```python
from build123d import *

# Parameters (mm, degrees)
SKETCH1_W           = 700
SKETCH1_H           = 50
SKETCH1_R           = 6
BOSS_EXTRUDE1_DEPTH = 10
FILLET1_RADIUS      = 25
FILLET1_LENGTH      = 10
FILLET2_RADIUS      = 25
FILLET2_LENGTH      = 10
BOSS_EXTRUDE2_DEPTH = 10
SKETCH3_R           = 100
SKETCH3_R_2         = 82.5
BOSS_EXTRUDE3_DEPTH = 30
SKETCH4_R           = 4.5
CUT_EXTRUDE1_DEPTH  = 815.631818676
CIRPATTERN1_COUNT   = 8


with BuildPart() as part:
    # Sketch1 → Boss-Extrude1 (new body)
    with BuildSketch(Plane.XY):
        Rectangle(SKETCH1_W, SKETCH1_H)
        with Locations((-300, 0)):
            Circle(SKETCH1_R, mode=Mode.SUBTRACT)
        with Locations((300, 0)):
            Circle(SKETCH1_R, mode=Mode.SUBTRACT)
    extrude(amount=BOSS_EXTRUDE1_DEPTH)

    # Fillet1: full round fillet: the end face becomes a half cylinder, R = half its width
    fillet1_face = Plane((-350, 0, 5), x_dir=(0, 0, 1), z_dir=(-1, 0, 0))  # on the end face: x along it, z out of the body
    fillet1_slab = fillet1_face.offset(-FILLET1_RADIUS / 2) * Box(FILLET1_LENGTH, 2 * FILLET1_RADIUS, FILLET1_RADIUS, mode=Mode.PRIVATE)  # the body's end, R deep
    fillet1_round = Plane((-325, 0, 5), x_dir=(-1, 0, 0), z_dir=(0, 0, 1)) * Cylinder(FILLET1_RADIUS, FILLET1_LENGTH, mode=Mode.PRIVATE)  # its axis R under the face
    add(fillet1_slab - fillet1_round, mode=Mode.SUBTRACT)

    # Fillet2: full round fillet: the end face becomes a half cylinder, R = half its width
    fillet2_face = Plane((350, 0, 5), x_dir=(0, 0, -1), z_dir=(1, 0, 0))  # on the end face: x along it, z out of the body
    fillet2_slab = fillet2_face.offset(-FILLET2_RADIUS / 2) * Box(FILLET2_LENGTH, 2 * FILLET2_RADIUS, FILLET2_RADIUS, mode=Mode.PRIVATE)  # the body's end, R deep
    fillet2_round = Plane((325, 0, 5), x_dir=(1, 0, 0), z_dir=(0, 0, -1)) * Cylinder(FILLET2_RADIUS, FILLET2_LENGTH, mode=Mode.PRIVATE)  # its axis R under the face
    add(fillet2_slab - fillet2_round, mode=Mode.SUBTRACT)

    # Sketch2 → Boss-Extrude2 (add)
    with BuildSketch(Plane.XY.offset(10)):
        Polygon((-325, 25), (-85, 735), (85, 735), (325, 25), align=None)
    extrude(amount=-BOSS_EXTRUDE2_DEPTH)

    # Sketch3 → Boss-Extrude3 (add)
    with BuildSketch(Plane.XY.offset(10)):
        with Locations(Location((0, 472, 0), (0, 0, 180))):
            Circle(SKETCH3_R)
        with Locations((0, 472)):
            Circle(SKETCH3_R_2, mode=Mode.SUBTRACT)
    extrude(amount=BOSS_EXTRUDE3_DEPTH)

    # Sketch4 → Cut-Extrude1 (cut, through all)
    with BuildSketch(Plane.XY.offset(10)):
        with Locations((-37.739196917, 413.044482735)):
            Circle(SKETCH4_R)
    cut_extrude1 = extrude(amount=-CUT_EXTRUDE1_DEPTH, mode=Mode.SUBTRACT)

    # CirPattern1: Cut-Extrude1 ×8 about axis
    cirpattern1_axis = Axis((0, 472, 0), (0, 0, 1))
    for i in range(1, CIRPATTERN1_COUNT):
        add(cut_extrude1.rotate(cirpattern1_axis, i * 360 / CIRPATTERN1_COUNT), mode=Mode.SUBTRACT)


solid = part.part
```
Here's how the part is built. I have some questions about the finished solid (model axes, mm). A direction names the side the tool comes from. Give positions to 0.01 mm unless a question says otherwise; leave off trailing zeros. Loops run counter-clockwise (first coordinate to the right, second up) from the corner with the lowest first, then second, coordinate; pieces in that order, holes last. Notation, with made-up numbers: M 63,5.5 L 106,5.5 A20 ccw 106,14.5 Z; hole C 61,-35.75 d9. An arc over 180 degrees is marked long. Put each result on its own line as item: value. Start each with the question number.
(1) I want a section at A-A on z = 26. Please give me the cut outline in (x, y).
(2) I need wall thicknesses on line 1 along Y through (x, z) = (-0.5, 35.5); line 2 along Z through (x, y) = (-76.5, 451); line 3 along Y through (x, z) = (27, 27.5). Which ranges of each line are inside material? Lowest first, please. Write a range as [from, to].
(3) I want a section at C-C on x = 276. Please give me the cut outline in (y, z), then the cut area to 3 significant figures.
(4) For faces 4 (the flat face through (5, 276, 0)), 5 (the cylindrical face through (38.07, 398.81, 24.79)), which set-ups out of +Z, -Z, +X, -X, +Y, -Y let a thin tool reach every point of the face, with its end or its side?
(5) Will these pins go through, and if not, where does the flat tip stop? pin 1 Ø15.5 at (x, y) = (-300, 0) entering from +Z; pin 2 Ø5 at (y, z) = (497.5, 15) entering from +X.
(6) I want a section at B-B on y = 594.5. Please give me the cut outline in (x, z).
(7) If we mould it in two halves opening along Y, with no side actions, what happens to faces 1 (the flat face through (1, 473, 10)), 2 (the flat face through (-14, 390, 40)), 3 (the cylindrical face through (349.994, 0.55, 4.93))? For each: +Y half, -Y half, draft (parallel to the pull), parting line (faces both ways), or undercut.
Answer block:
1. outline: C 0,472 d200; hole C 0,472 d165
2. line 1: [372, 389.5], [554.5, 572]
2. line 2: [0, 10]
2. line 3: [375.71, 394.04], [549.96, 568.29]
3. outline: M -25,0 L 169.96,0 L 169.96,10 L -25,10 Z
3. area: 1,950 mm^2
4. face 4: -Z, +X, -X, +Y, -Y
4. face 5: +Z
5. pin 1: z = 10
5. pin 2: x = 97.32
6. outline: M -132.49,0 L 132.49,0 L 132.49,10 L -132.49,10 Z
7. face 1: undercut
7. face 2: draft
7. face 3: parting line
